Study the drawing (mm; zero at the part's minimum x, y, z) and answer. A direction names the side the tool comes from. Coordinates: 2 decimals unless noted, no trailing zeros. Loops run counter-clockwise (first coordinate to the right, second up) from the corner with the lowest first, then second, coordinate; pieces in that order, holes last. Notation, with made-up numbers: (-16.5, 44.5) - (24.5, 44.5) arc R22 ccw to (24.5, 72.5) - close; hole circle Ø9 at (-10, 59). An arc over 180 degrees is marked (long way). Use one line per item in the form item = value.
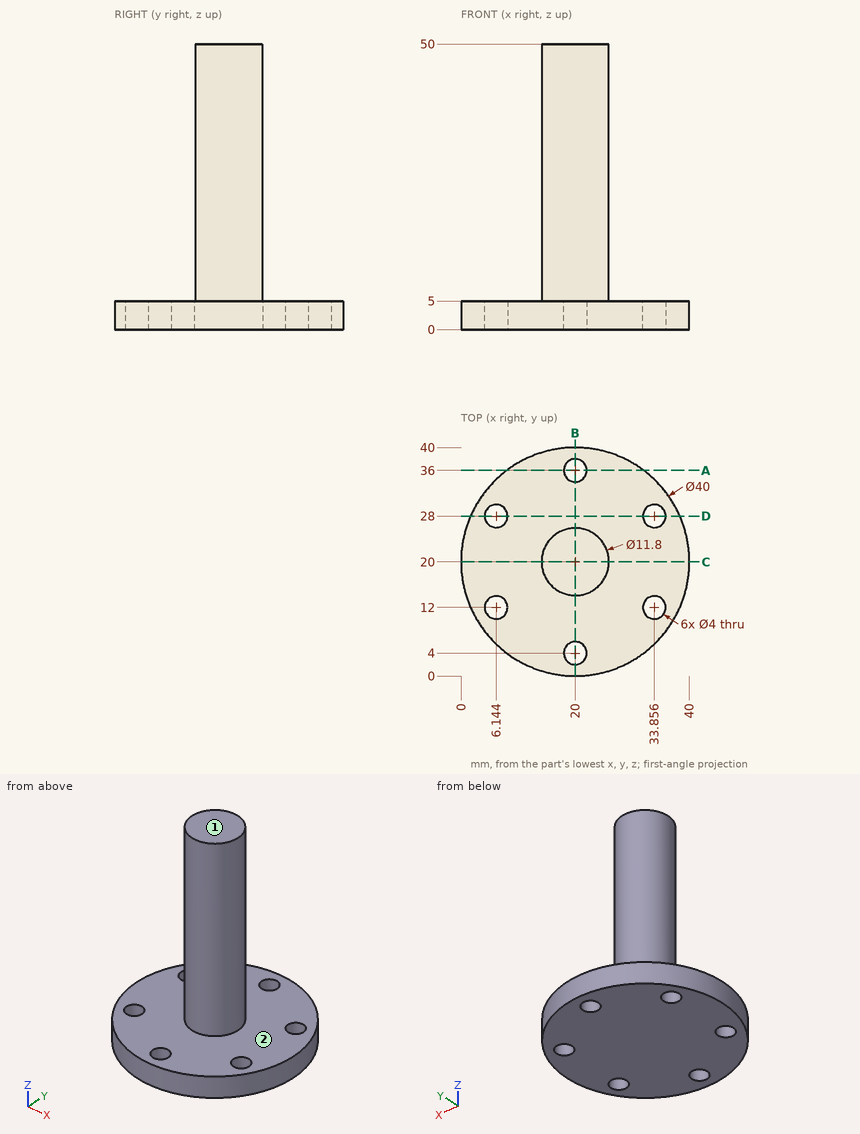
Item 1: The part is cut by section B-B on x = 20. Give the vertices of the cut face in (y, z), plus the area to 3 significant figures.
Results below:
outline = (0, 0) - (2, 0) - (2, 5) - (0, 5) - close; (6, 0) - (34, 0) - (34, 5) - (25.9, 5) - (25.9, 50) - (14.1, 50) - (14.1, 5) - (6, 5) - close; (38, 0) - (40, 0) - (40, 5) - (38, 5) - close
area = 691 mm²
Item 2: The part is cut by section D-D on y = 28. Give the vertices of the cut face in (x, z), plus the area to 3 significant figures.
Results below:
outline = (1.67, 0) - (4.14, 0) - (4.14, 5) - (1.67, 5) - close; (8.14, 0) - (31.86, 0) - (31.86, 5) - (8.14, 5) - close; (35.86, 0) - (38.33, 0) - (38.33, 5) - (35.86, 5) - close
area = 143 mm²
Item 3: The part is cut by section A-A on y = 36. Give the vertices of the cut face in (x, z).
Results below:
outline = (8, 0) - (18, 0) - (18, 5) - (8, 5) - close; (22, 0) - (32, 0) - (32, 5) - (22, 5) - close
Item 4: Each of these flat-tipped pins is pushed along its axis until it touches: P1, Ø3, axis at y = 17.5, z = 34.5, coming from the +X side (1 decimal); P2, Ø5, axis at x = 33.86, y = 12, coming from the -Z side; P3, Ø6.5, axis at x = 33.86, y = 28, coming from the +Z side; P4, Ø4, axis at y = 13, z = 22, coming from the +X side. Where does it stop, or does it pass through?
Results below:
P1 = 25.8
P2 = 0
P3 = 5
P4 = 23.13
Item 5: Find the intervals of material crossed by L1, parallel to Y at x = 20, z = 2.4; L2, parallel to Z at x = 19.5, y = 12; L3, parallel to Y at x = 19, z = 39.5 (1 decimal), in increasing order.
Results below:
L1 = 0 to 2, 6 to 34, 38 to 40
L2 = 0 to 5
L3 = 14.2 to 25.8
Item 6: The part is cut by section C-C on y = 20. Give the vertices of the cut face in (x, z), plus the area to 3 significant figures.
Results below:
outline = (0, 0) - (40, 0) - (40, 5) - (25.9, 5) - (25.9, 50) - (14.1, 50) - (14.1, 5) - (0, 5) - close
area = 731 mm²
Item 7: Which of the six approach directions +Z, -Z, +X, -X, +Y, -Y give full straight-line access (tool end or side, diameter ignored) to the marked faces 1 and 2?
Results below:
face_1 = +Z, +X, -X, +Y, -Y
face_2 = +Z
